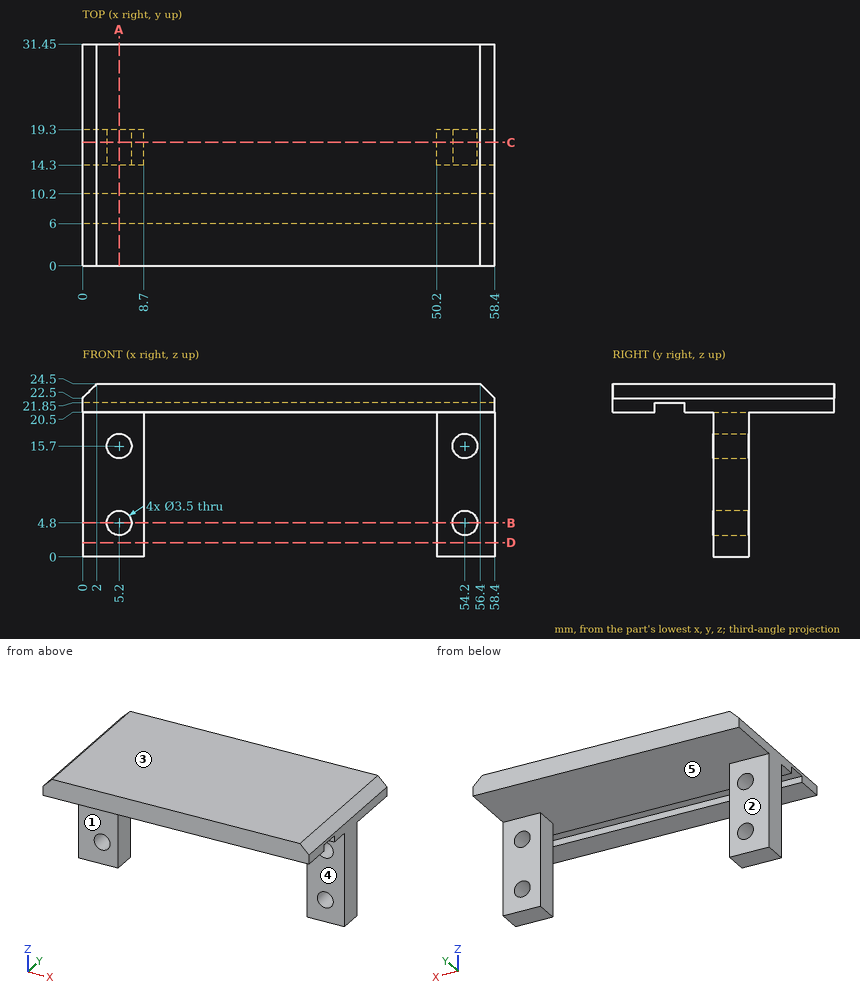
Here's the drawing with two shaded views (mm, measured from the low corner). I have some questions. A direction names the side the tool comes from. Coordinates: 2 decimals unless noted, no trailing zeros. Write each loop counter-clockwise with the first axis right and the second up, starting at its lowest first coordinate (ties: lowest second). Pieces come first, ordered by that corner, then holes. Notation, with made-up numbers: M -29.5,68.5 L 26.5,68.5 A24 cw 26.5,81.5 Z; hole C 24.5,-22.5 d1. An arc over 180 degrees is marked long. Answer as CSV lines item,"result". Start each with the question number.
1) We'd pull the mould along X, two halves only. Please class the marked faces 4 and 5: +X half, -X half, draft (parallel to the pull), parting line (faces both ways), or undercut.
2) I want a section at B-B, the plane z = 4.8. Please give me the cut outline in (x, y).
3) Please list where these lines run through material, in increasing order: line 1 (Y direction, x = 27, z = 21.5); line 2 (X direction, y = 16, z = 13); line 3 (Z direction, x = 19, y = 11). Write a range as from..to.
4) I want a section at A-A, the plane x = 5.2. Please give me the cut outline in (y, z).
5) I want a section at D-D, the plane z = 2. Please give me the cut outline in (x, y), and give its area (3 significant figures).
6) For the marked faces 1, 2 and 3, which set-ups out of +Z, -Z, +X, -X, +Y, -Y let a thin tool reach every point of the face, with its end or its side?
7) For P1, Ø17, axis at x = 19.5, y = 17, coming from the -Z side; P2, Ø7, axis at x = 3, z = 9, coming from the +Y side; P3, Ø4, axis at x = 54.2, z = 15.7, coming from the -Y side, each with a flat end and sliding along its axis, tell me the tip position at first contact or that it passes through.
8) I want a section at C-C, the plane y = 17.5. Please give me the cut outline in (x, z).
Data:
1,face 4,"draft"
1,face 5,"undercut"
2,outline,"M 0,14.3 L 3.45,14.3 L 3.45,19.3 L 0,19.3 Z; M 6.95,14.3 L 8.7,14.3 L 8.7,19.3 L 6.95,19.3 Z; M 50.2,14.3 L 52.45,14.3 L 52.45,19.3 L 50.2,19.3 Z; M 55.95,14.3 L 58.4,14.3 L 58.4,19.3 L 55.95,19.3 Z"
3,line 1,"y = 0..6, 10.2..31.45"
3,line 2,"x = 0..8.7, 50.2..58.4"
3,line 3,"z = 20.5..24.5"
4,outline,"M 0,20.5 L 6,20.5 L 6,21.85 L 10.2,21.85 L 10.2,20.5 L 14.3,20.5 L 14.3,17.45 L 19.3,17.45 L 19.3,20.5 L 31.45,20.5 L 31.45,24.5 L 0,24.5 Z; M 14.3,0 L 19.3,0 L 19.3,3.05 L 14.3,3.05 Z; M 14.3,6.55 L 19.3,6.55 L 19.3,13.95 L 14.3,13.95 Z"
5,outline,"M 0,14.3 L 8.7,14.3 L 8.7,19.3 L 0,19.3 Z; M 50.2,14.3 L 58.4,14.3 L 58.4,19.3 L 50.2,19.3 Z"
5,area,"84.5 mm^2"
6,face 1,"-Z, +X, -X, -Y"
6,face 2,"-Z, +X, -X, +Y"
6,face 3,"+Z, +X, -X, +Y, -Y"
7,P1,"stops at z = 20.5"
7,P2,"stops at y = 19.3"
7,P3,"stops at y = 14.3"
8,outline,"M 0,0 L 8.7,0 L 8.7,20.5 L 50.2,20.5 L 50.2,0 L 58.4,0 L 58.4,22.5 L 56.4,24.5 L 2,24.5 L 0,22.5 Z; hole C 5.2,4.8 d3.5; hole C 5.2,15.7 d3.5; hole C 54.2,4.8 d3.5; hole C 54.2,15.7 d3.5"
